Here's how the part is built. I have some questions about the finished solid (model axes, mm). A direction names the side the tool comes from. Round coordinates to 2 decimals unless told otherwise and drop trailing zeros. Order: outer loops, then holes, each group sorted by start corner. A loop starts at its lowest first (then second) coordinate and runs counter-clockwise, first axis right, second up. Notation, with made-up numbers: (8, 70.5) - (50, 70.5) arc R14 cw to (50, 96.5) - close; hole circle Ø9 at (6, 21). An arc over 180 degrees is marked (long way). Answer as a JSON object with one key per item and string values.
```python
from build123d import *

# Parameters (mm, degrees)
F1_DEPTH = 152.4
F2_R     = 15.9434663659


# Not quite as in the source:
# - a feature names something its author has since deleted; it is built from what else it names


with BuildPart() as f1:
    # F0 (on Front) → F1 (new body)
    with BuildSketch(Plane.XZ):
        Polygon((-233.7148142715, -101.2738309481), (-233.7148142715, -149.9473750383), (71.0851857285, -149.9473750383), (71.0851857285, 44.3499535322), (71.0851857285, 88.5266363621), (4.2222592115, 154.8526249617), (-173.5777407885, 154.8526249617), (-233.7148142715, 89.2168954015), (-220.7819144912, 77.3674537994), (-233.7148142715, 63.2520294323), (-220.7819144912, 51.4025878302), (-233.7148142715, 40.2083918452), (-221.5843061602, 22.7510556579), (-233.7148142715, 13.7644242495), (-223.5177305101, 0), (-233.7148142715, -7.5542947057), (-223.5177305101, -21.3187189553), (-233.7148142715, -37.3470336199), (-223.5177305101, -43.8343355859), (-233.7148142715, -54.8694915965), (-220.7819144912, -66.8201937171), (-233.7148142715, -80.8160154721), (-223.5177305101, -90.2386749375), align=None)
    extrude(amount=F1_DEPTH)

    # F2
    f2_edges = [f1.edges().sort_by_distance(p)[0] for p in [
        (-84.677741, -152.4, 154.852625),
        (-84.677741, 0, 154.852625),
    ]]
    fillet(f2_edges, radius=F2_R)


solid = f1.part
```
1. If I drill on L1, parallel to Z at x = 7.5, y = -47.5; L2, parallel to X at y = -53.5, z = 80; L3, parallel to X at y = -63.5, z = 5, over which ranges is the centre line in solid material (lowest first)? Write a range as [from, to].
Responses:
{"L1": "[-149.95, 151.6]", "L2": "[-223.66, 71.09]", "L3": "[-227.22, 71.09]"}
2. Imagine slicing it at A-A (y = -32). List the corners of the cut face in (x, z) for me, plus the area to 3 significant figures.
Responses:
{"outline": "(-233.71, -149.95) - (71.09, -149.95) - (71.09, 88.53) - (4.22, 154.85) - (-173.58, 154.85) - (-233.71, 89.22) - (-220.78, 77.37) - (-233.71, 63.25) - (-220.78, 51.4) - (-233.71, 40.21) - (-221.58, 22.75) - (-233.71, 13.76) - (-223.52, 0) - (-233.71, -7.55) - (-223.52, -21.32) - (-233.71, -37.35) - (-223.52, -43.83) - (-233.71, -54.87) - (-220.78, -66.82) - (-233.71, -80.82) - (-223.52, -90.24) - (-233.71, -101.27) - close", "area": "87,600 mm2"}
3. For P1, Ø3, axis at y = -119, z = 12, coming from the -X side; P2, Ø10, axis at y = -27.5, z = -91.5, coming from the -X side, each with a flat end and sliding along its axis, tell me the tip position at first contact or that it passes through.
Responses:
{"P1": "x = -233.52", "P2": "x = -229.3"}
4. Thinking about a two-plate mould opening in Z: for faces 3 (the face through (-227.339, -75.133, 83.375)), 4 (the face through (-83, 0, -3)), 5 (the face through (-85.405, -4.794, 150.306)), which applies, pulls with the +Z half, pulls with the -Z half, needs draft (parallel to the pull), parting line crosses it, or undercut?
Responses:
{"face 3": "undercut", "face 4": "needs draft", "face 5": "pulls with the +Z half"}
5. For faces 1 (the face through (38.122, -75.133, 121.225)), 2 (the face through (-228.54, -75.13, -49.27)), which set-ups out of +Z, -Z, +X, -X, +Y, -Y let a thin tool reach every point of the face, with its end or its side?
Responses:
{"face 1": "+Z, +X, +Y, -Y", "face 2": "-X, +Y, -Y"}
6. Imagine slicing it at B-B (z = 130). List the corners of the cut face in (x, y) for me.
Responses:
{"outline": "(-196.35, -152.4) - (29.28, -152.4) - (29.28, 0) - (-196.35, 0) - close"}
